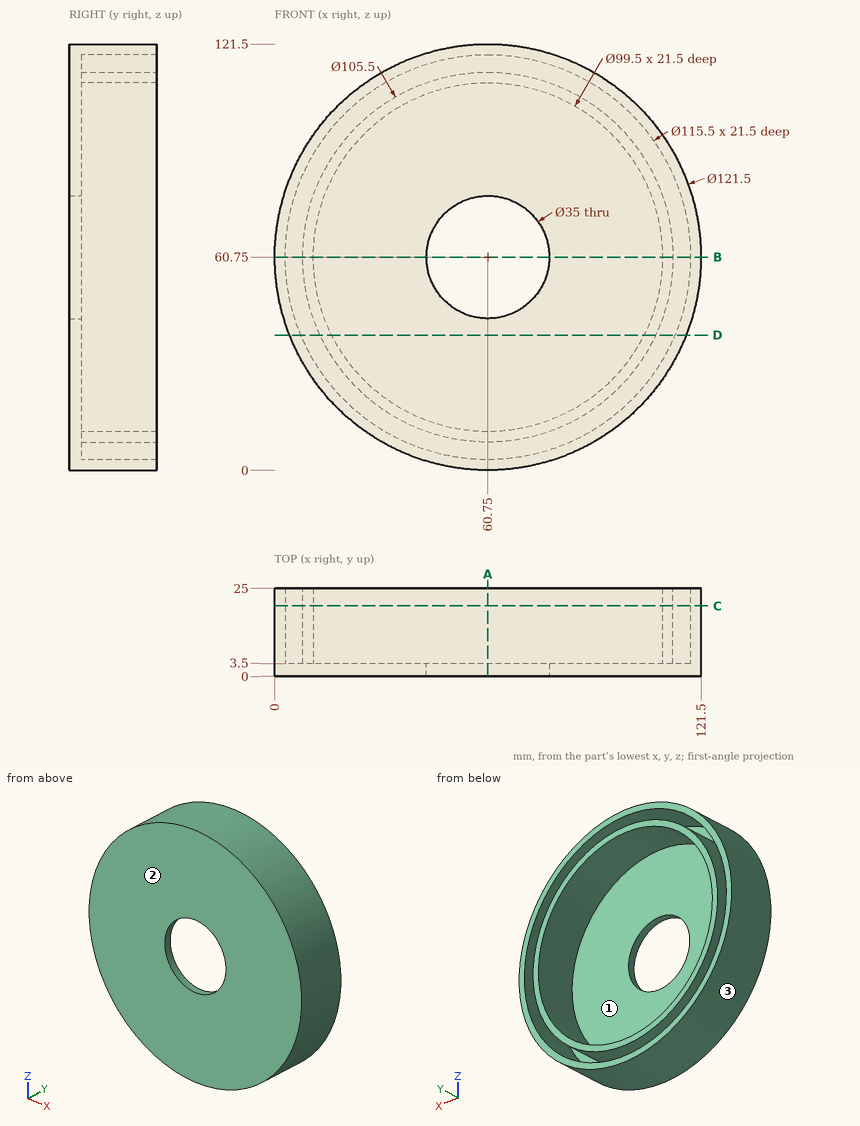
Print and shaded views of the part. All mm, measured from the part's lowest x, y and z. Coordinates: 2 decimals unless noted, no trailing zeros. Loops run counter-clockwise (first coordinate to the right, second up) from the corner with the lowest first, then second, coordinate; pieces in that order, holes last. Notation, with made-up numbers: M -28,-20.75 L 18,-20.75 A21 ccw 18,-9.75 Z; hole C 37.5,60.25 d3. An arc over 180 degrees is marked long. Use a Markdown table: item, result. Add a question column.
Q1. Probe L1, parallel to X at y = 17.5, z = 60.75; L2, parallel to X at y = 2.2, z = 60.75; L3, parallel to Z at x = 73, y = 12.5. List the from-to ranges inside material, lowest first.
Q2. Cut at C-C (y = 20). Write the cut outline in (x, z), and give its area (3 significant figures).
Q3. Cut at D-D (z = 38.5). Write the cut outline in (x, y).
Q4. Pin check, flat tips, straight feed: P1, Ø4, axis at x = 80, z = 36, coming from the +Y side; P2, Ø1.5, axis at y = 11, z = 94.5, coming from the -X side; P3, Ø4, axis at y = 14.5, z = 45, coming from the +X side. Stop position of each tip, or through.
Q5. Cut at B-B (z = 60.75). Write the cut outline in (x, y), and give its area (3 significant figures).
Q6. Cut at A-A (x = 60.75). Write the cut outline in (y, z).
Q7. Mould opens along Z. For the marked faces 1, 2 and 3 say: +Z half, -Z half, draft (parallel to the pull), parting line (faces both ways), or undercut.
Worked out:
| question | item | result |
|---|---|---|
| 1 | L1 | x = 0 to 3, 8 to 11, 110.5 to 113.5, 118.5 to 121.5 |
| 1 | L2 | x = 0 to 43.25, 78.25 to 121.5 |
| 1 | L3 | z = 1.25 to 4.31, 9.44 to 12.53, 108.97 to 112.06, 117.19 to 120.25 |
| 2 | outline | C 60.75,60.75 d121.5; C 60.75,60.75 d105.5; hole C 60.75,60.75 d115.5; hole C 60.75,60.75 d99.5 |
| 2 | area | 2,080 mm2 |
| 3 | outline | M 4.22,0 L 117.28,0 L 117.28,25 L 114.04,25 L 114.04,3.5 L 108.58,3.5 L 108.58,25 L 105.25,25 L 105.25,3.5 L 16.25,3.5 L 16.25,25 L 12.92,25 L 12.92,3.5 L 7.46,3.5 L 7.46,25 L 4.22,25 Z |
| 4 | P1 | stops at y = 3.5 |
| 4 | P2 | stops at x = 9.74 |
| 4 | P3 | stops at x = 119.92 |
| 5 | outline | M 0,0 L 43.25,0 L 43.25,3.5 L 11,3.5 L 11,25 L 8,25 L 8,3.5 L 3,3.5 L 3,25 L 0,25 Z; M 78.25,0 L 121.5,0 L 121.5,25 L 118.5,25 L 118.5,3.5 L 113.5,3.5 L 113.5,25 L 110.5,25 L 110.5,3.5 L 78.25,3.5 Z |
| 5 | area | 561 mm2 |
| 6 | outline | M 0,0 L 25,0 L 25,3 L 3.5,3 L 3.5,8 L 25,8 L 25,11 L 3.5,11 L 3.5,43.25 L 0,43.25 Z; M 0,78.25 L 3.5,78.25 L 3.5,110.5 L 25,110.5 L 25,113.5 L 3.5,113.5 L 3.5,118.5 L 25,118.5 L 25,121.5 L 0,121.5 Z |
| 7 | face 1 | undercut |
| 7 | face 2 | draft |
| 7 | face 3 | parting line |
